from build123d import *

# Parameters (mm, degrees)
SKETCH1_W           = 229.859874896
SKETCH1_H           = 171.45
BOSS_EXTRUDE1_DEPTH = 6.35
SKETCH2_W           = 25.4
SKETCH2_H           = 6.35
CUT_EXTRUDE1_DEPTH  = 6.35
LPATTERN1_COUNT     = 4
LPATTERN1_PITCH     = 50.8
SKETCH4_R           = 2.0955
CUT_EXTRUDE2_DEPTH  = 209.955242778
SKETCH5_W           = 25.4
SKETCH5_H           = 6.35
SKETCH5_W_2         = 25.290516307
SKETCH5_W_3         = 6.35
SKETCH5_H_2         = 25.4
CUT_EXTRUDE3_DEPTH  = 6.35


with BuildPart() as part:
    # Sketch1 → Boss-Extrude1 (new body)
    with BuildSketch(Plane.XY):
        with Locations((-24.419947229, 69.85)):
            Rectangle(SKETCH1_W, SKETCH1_H)
    extrude(amount=BOSS_EXTRUDE1_DEPTH)

    # Sketch2 → Cut-Extrude1 (cut)
    with BuildSketch(Plane.XY.offset(6.35)):
        with Locations((-99.990009781, -12.7)):
            Rectangle(SKETCH2_W, SKETCH2_H)
        with Locations((-99.990009781, 152.4)):
            Rectangle(SKETCH2_W, SKETCH2_H)
    cut_extrude1 = extrude(amount=-CUT_EXTRUDE1_DEPTH, mode=Mode.SUBTRACT)

    # LPattern1: Cut-Extrude1 ×4
    with Locations(*[(i * LPATTERN1_PITCH, 0, 0) for i in range(1, LPATTERN1_COUNT)]):
        add(cut_extrude1, mode=Mode.SUBTRACT)

    # Sketch4 → Cut-Extrude2 (cut, through all)
    with BuildSketch(Plane(origin=(0, 0, 0), x_dir=(-1, 0, 0), z_dir=(0, 0, -1))):
        with Locations((-77.809990219, -12.7)):
            Circle(SKETCH4_R)
        with Locations((23.790009781, -12.7)):
            Circle(SKETCH4_R)
        with Locations((126.019947229, -12.7)):
            Circle(SKETCH4_R)
        with Locations((126.019947229, 152.4)):
            Circle(SKETCH4_R)
        with Locations((23.790009781, 152.4)):
            Circle(SKETCH4_R)
        with Locations((-77.809990219, 152.4)):
            Circle(SKETCH4_R)
    extrude(amount=-CUT_EXTRUDE2_DEPTH, mode=Mode.SUBTRACT)

    # Sketch5 → Cut-Extrude3 (cut)
    with BuildSketch(Plane(origin=(0, 0, 0), x_dir=(-1, 0, 0), z_dir=(0, 0, -1))):
        with Locations((-39.709990219, 4.7625)):
            Rectangle(SKETCH5_W, SKETCH5_H)
        with Locations((11.035267935, 4.7625)):
            Rectangle(SKETCH5_W_2, SKETCH5_H)
        with Locations((61.890009781, 4.7625)):
            Rectangle(SKETCH5_W, SKETCH5_H)
        with Locations((103.165009781, 39.6875)):
            Rectangle(SKETCH5_W_3, SKETCH5_H_2)
        with Locations((103.165009781, 103.1875)):
            Rectangle(SKETCH5_W_3, SKETCH5_H_2)
        with Locations((61.890009781, 134.9375)):
            Rectangle(SKETCH5_W, SKETCH5_H)
        with Locations((11.090009781, 134.9375)):
            Rectangle(SKETCH5_W, SKETCH5_H)
        with Locations((-39.709990219, 134.9375)):
            Rectangle(SKETCH5_W, SKETCH5_H)
    extrude(amount=-CUT_EXTRUDE3_DEPTH, mode=Mode.SUBTRACT)


solid = part.part
The model under review builds one solid part; all positions refer to its coordinate system, in mm. A direction names the side the tool comes from. Round coordinates to 2 decimals unless told otherwise and drop trailing zeros. Loops run counter-clockwise (first coordinate to the right, second up) from the corner with the lowest first, then second, coordinate; pieces in that order, holes last. Notation, with made-up numbers: (-3, 63) -> (10, 63) arc R21 ccw to (10, 81) -> close; hole circle Ø4 at (7.5, 65.25). An arc over 180 degrees is marked (long way). One line per question, with ' | ' between items. Start each with the question number.
Item 1: Draft analysis for pull direction X (two halves, no side actions). For faces 4 (the face through (40, 138.112, 3)), 5 (the face through (-139.35, 69, 3)), 6 (the face through (-24, 155.575, 3)), state which applies: +X half, -X half, draft (parallel to the pull), parting line (faces both ways), or undercut.
Item 2: For pin 1 (1.9 mm diameter, centred on x = -45.5, z = 4, fed in from -Y) (3 decimals), flat-tipped, find the tip position at first contact; note if it passes through.
Item 3: Add section B-B, the plane x = -109. Write out the cut boundary in (y, z) (3 decimals).
Item 4: Machinability: for faces 1 (the face through (40, 7.938, 3)), 2 (the face through (-11.09, 152, 3)), 3 (the face through (1, -9.525, 3)), which of the approach directions +Z, -Z, +X, -X, +Y, -Y give a long, thin tool a straight path to every point of the face, cutting with its end or side? Answer none if there is none.
Item 5: Wall thickness on line 1 along X through (y, z) = (132, 4.75); line 2 along Y through (x, z) = (31.5, 0.75) (1 decimal); line 3 along Y through (x, z) = (-57, 4.25) (1 decimal): over which ranges is each line inside the solid? List them lowest first. Write a range as [from, to].
Item 6: Add section A-A, the plane x = 46.5. Count the separate pieces of the cut face and the enclosed holes in it, then the cut area to 3 significant figures.
Return value:
1) face 4: undercut | face 5: -X half | face 6: draft
2) pin 1: stops at y = -9.525
3) outline: (-9.525, 0) -> (149.225, 0) -> (149.225, 6.35) -> (-9.525, 6.35) -> close
4) face 1: +Z, -Z | face 2: +Z, -Z, +Y | face 3: +Z, -Z, -Y
5) line 1: x = [-139.35, -74.59], [-49.19, -23.79], [1.61, 27.01], [52.41, 90.51] | line 2: y = [-15.9, 1.6], [7.9, 131.8], [138.1, 155.6] | line 3: y = [-9.5, 1.6], [7.9, 131.8], [138.1, 149.2]
6) separate pieces: 3 | enclosed holes: 0 | area: 927 mm2
